Build history of the part. All positions in model axes, mm. Face numbers are marked on the shaded views. A direction names the side the tool comes from. Round coordinates to 2 decimals unless told otherwise and drop trailing zeros. Order: outer loops, then holes, each group sorted by start corner. A loop starts at its lowest first (then second) coordinate and runs counter-clockwise, first axis right, second up. Notation, with made-up numbers: (9.5, -10) - (34.5, -10) arc R27 ccw to (34.5, 16) - close; hole circle Ø3 at (-28.75, 23.25). An arc over 180 degrees is marked (long way). One line per question, with ' | ' between items. Start each with the question number.
Autodesk Inventor part; units mm, degrees
ref_plane "YZ Plane" through (0, 0, 0) normal (1, 0, 0) x (0, 1, 0)
ref_plane "XZ Plane" through (0, 0, 0) normal (0, 1, 0) x (-1, 0, 0)
ref_plane "XY Plane" through (0, 0, 0) normal (0, 0, 1) x (1, 0, 0)
sketch "Sketch1" plane through (0, 0, 0) normal (0, 0, 1) x (1, 0, 0)
  circle A0 centre (0, 0) radius 2
  circle A1 centre (0, 17.3205) radius 2
  circle A2 centre (-15, -8.6603) radius 2
  circle A3 centre (15, -8.6603) radius 2
  line L0 (-15, -16.1603) -> (15, -16.1603)
  line L1 (21.4952, -4.9103) -> (6.4952, 21.0705)
  line L2 (-6.4952, 21.0705) -> (-21.4952, -4.9103)
  arc A4 (6.4952, 21.0705) -> (-6.4952, 21.0705) centre (0, 17.3205) ccw
  arc A5 (15, -16.1603) -> (21.4952, -4.9103) centre (15, -8.6603) ccw
  arc A6 (-21.4952, -4.9103) -> (-15, -16.1603) centre (-15, -8.6603) ccw
  line L3 (15.512, -26.8675) -> (-15.512, -26.8675)
  line L4 (15.512, 26.8675) -> (31.0239, 0)
  line L5 (-31.0239, 0) -> (-15.512, 26.8675)
  line L6 (-31.0239, 0) -> (-15.512, -26.8675)
  line L7 (15.512, -26.8675) -> (31.0239, 0)
  line L8 (15.512, 26.8675) -> (-15.512, 26.8675)
  point P0 (0, 0)
  dimension "d3" = 7.5
extrude "Extrusion1" add sketch "Sketch1" along normal blind 10 contours A0 | A1 | A2 | A3 | A6 L2 A4 L1 A5 L0
sketch "Sketch2" plane through (0, 0, 0) normal (0, 0, -1) x (-1, 0, 0)
  arc A0 (15, -16.1603) -> (21.4952, -4.9103) centre (15, -8.6603) ccw
  arc A1 (6.4952, 21.0705) -> (-6.4952, 21.0705) centre (0, 17.3205) ccw
  arc A2 (-21.4952, -4.9103) -> (-15, -16.1603) centre (-15, -8.6603) ccw
  point P0 (0, 0)
hole "Hole1" at (0, 17.3205, 0) at (15, -8.6603, 0) at (-15, -8.6603, 0) direction (0, 0, 1) diameter 4.5 depth 5.25
sketch "Sketch3" plane through (0, 0, 0) normal (0, 0, -1) x (-1, 0, 0)
  point P0 (0, 0)
hole "Hole2" at (0, 0, 0) direction (0, 0, 1) diameter 3 end through all
sketch "Sketch4" plane through (0, 0, 10) normal (0, 0, 1) x (1, 0, 0)
  arc A0 (15, -16.1603) -> (21.4952, -4.9103) centre (15, -8.6603) ccw
  arc A1 (6.4952, 21.0705) -> (-6.4952, 21.0705) centre (0, 17.3205) ccw
  arc A2 (-21.4952, -4.9103) -> (-15, -16.1603) centre (-15, -8.6603) ccw
  circle A3 centre (0, 17.3205) radius 7.5
  circle A4 centre (15, -8.6603) radius 7.5
  circle A5 centre (-15, -8.6603) radius 7.5
extrude "Extrusion2" add sketch "Sketch4" along normal blind 5
chamfer "Chamfer1" distance 2 angle 45 3 edges at (-22.5, -8.6603, 15) (-7.5, 17.3205, 15) (7.5, -8.6603, 15)
hole "Hole3" at (0, 17.3205, 15) direction (0, 0, -1) diameter 3.5 depth 6
hole "Hole4" at (15, -8.6603, 15) direction (0, 0, -1) diameter 3.5 depth 6
hole "Hole5" at (-15, -8.6603, 15) direction (0, 0, -1) diameter 3.5 depth 6
properties part number "ShellFrame"
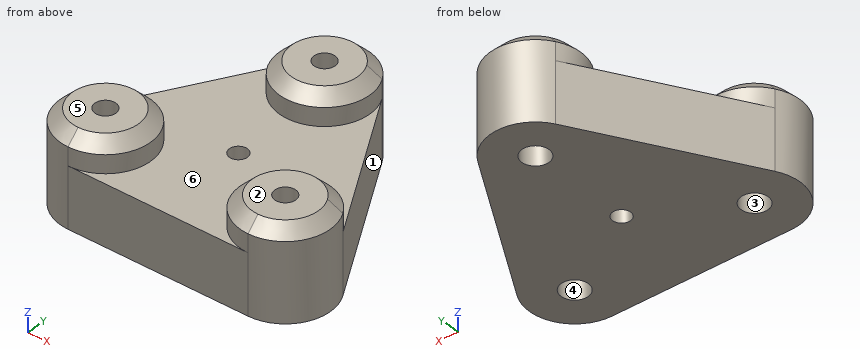
Item 1: Pull direction Y, two halves, no side cores. Call the marked faces 1, 2 and 3: released by +Y, released by -Y, zero draft, split by the parting line, or undercut.
Item 2: Slice it at A-A (x = 0). Write the cut outline in (y, z).
Item 3: Pin check, flat tips, straight feed: pin 1 (3 mm diameter, centred on x = 15, y = -8.66, fed in from +Z); pin 2 (1.3 mm diameter, centred on x = 15, y = -9.5, fed in from -Z); pin 3 (3 mm diameter, centred on x = -16, z = 8, fed in from +Y); pin 4 (2.5 mm diameter, centred on x = 0, y = 0, fed in from +Z). Stop position of each tip, or through.
Item 4: 3-axis set-ups, long thin cutter, end or side, ignore diameter. For the marked faces 4, 5 and 6: which of +Z, -Z, +X, -X, +Y, -Y reach the whole face in a straight line?
Item 5: Wall check: line 1 along Y through (x, z) = (0, 5); line 2 along Y through (x, z) = (2, 1.75); line 3 along X through (y, z) = (-5, 11.5). Give the ranges that are in metal, low to high. Write a range as [from, to].
Item 6: Slice it at C-C (y = 5.5). Write the cut outline in (x, z), plus the area to 3 significant figures.
Item 7: Slice it at B-B (y = 0). Write the cut outline in (x, z).
A:
1) face 1: released by +Y | face 2: zero draft | face 3: undercut
2) outline: (-16.16, 0) - (-1.5, 0) - (-1.5, 10) - (-16.16, 10) - close; (1.5, 0) - (15.07, 0) - (15.07, 5.25) - (19.57, 5.25) - (19.57, 0) - (24.82, 0) - (24.82, 13) - (22.82, 15) - (19.07, 15) - (19.07, 9) - (15.57, 9) - (15.57, 15) - (11.82, 15) - (9.82, 13) - (9.82, 10) - (1.5, 10) - close
3) pin 1: z = 9 | pin 2: z = 5.25 | pin 3: y = 7.21 | pin 4: through
4) face 4: -Z | face 5: +Z, +X, -X, +Y, -Y | face 6: +Z
5) line 1: [-16.16, -1.5], [1.5, 15.07], [19.57, 24.82] | line 2: [-16.16, 16.29], [18.35, 24.55] | line 3: [-21.55, -8.45], [8.45, 21.55]
6) outline: (-15.48, 0) - (15.48, 0) - (15.48, 10) - (-15.48, 10) - close | area: 310 mm^2
7) outline: (-18.66, 0) - (-1.5, 0) - (-1.5, 10) - (-18.66, 10) - close; (1.5, 0) - (18.66, 0) - (18.66, 10) - (1.5, 10) - close
